For this review, use the dimensioned drawing (mm, ordinates from the lowest corner) and the shaded views. Round coordinates to 2 decimals unless told otherwise and drop trailing zeros. Order: outer loops, then holes, each group sorted by start corner. A loop starts at its lowest first (then second) coordinate and runs counter-clockwise, first axis right, second up. Notation, with made-up numbers: (-3, 50) -> (10, 50) arc R18 cw to (10, 57) -> close; hole circle Ø11 at (-10.75, 18.25). An arc over 180 degrees is marked (long way). Use a Markdown table: item, result. Add a question column.
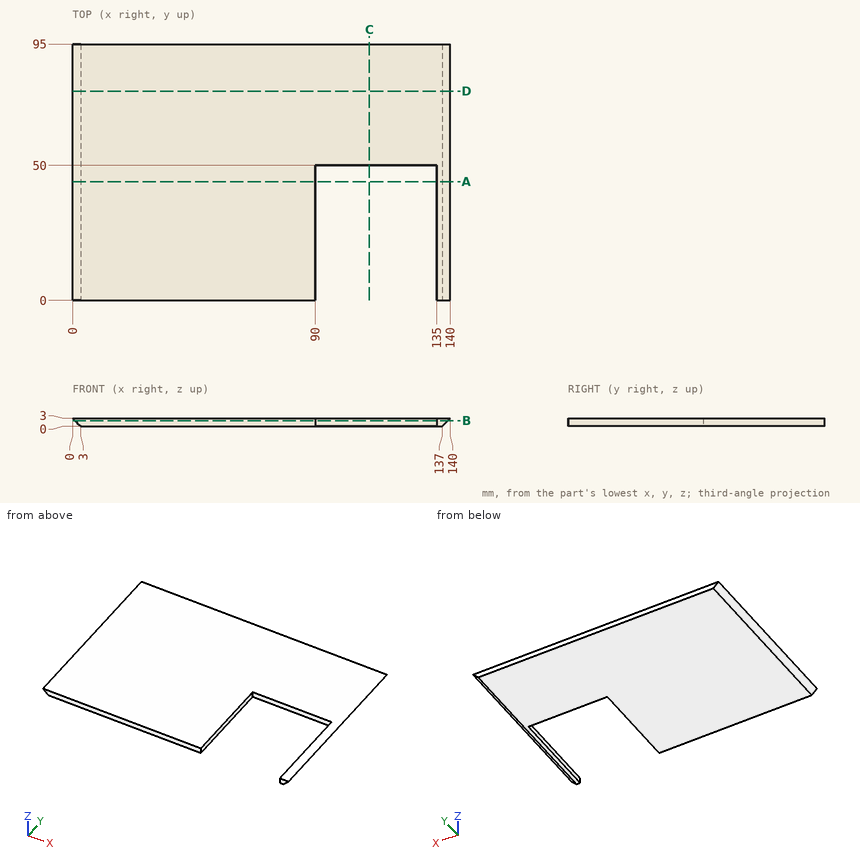
Q1. Add section B-B (z = 2.15). Write out the cut boundary in (x, y), then the cut area to 3 significant figures.
Q2. Add section D-D (y = 77.5). Write out the cut boundary in (x, z), then the cut area to 3 significant figures.
Q3. Insertion check: pin 1 (1.5 mm diameter, centred on x = 115, z = 1, fed in from -Y); pin 2 (0.9 mm diameter, centred on y = 16.5, z = 2, fed in from +X). Each pin has a flat end and moves straight along its axis. Give the tip position at first contact, or say it passes through.
Q4. Wall thickness on line 1 (Y direction, x = 91.5, z = 1.05); line 2 (X direction, y = 39.5, z = 0.3); line 3 (X direction, y = 20.5, z = 2.25): over which ranges is each line inside the solid? List them lowest first. Write a range as [from, to].
Q5. Add section C-C (x = 110). Write out the cut boundary in (y, z), then the cut area to 3 significant figures.
Q6. Add section A-A (y = 44). Write out the cut boundary in (x, z), then the cut area to 3 significant figures.
Report:
| question | item | result |
|---|---|---|
| 1 | outline | (0.85, 0) -> (90, 0) -> (90, 50) -> (135, 50) -> (135, 0) -> (139.15, 0) -> (139.15, 95) -> (0.85, 95) -> close |
| 1 | area | 10,900 mm² |
| 2 | outline | (0, 3) -> (3, 0) -> (137, 0) -> (140, 3) -> close |
| 2 | area | 411 mm² |
| 3 | pin 1 | stops at y = 50 |
| 3 | pin 2 | stops at x = 139.45 |
| 4 | line 1 | y = [50, 95] |
| 4 | line 2 | x = [2.7, 90], [135, 137.3] |
| 4 | line 3 | x = [0.75, 90], [135, 139.25] |
| 5 | outline | (50, 0) -> (95, 0) -> (95, 3) -> (50, 3) -> close |
| 5 | area | 135 mm² |
| 6 | outline | (0, 3) -> (3, 0) -> (90, 0) -> (90, 3) -> close; (135, 0) -> (137, 0) -> (140, 3) -> (135, 3) -> close |
| 6 | area | 276 mm² |
